from build123d import *

# Parameters (mm, degrees)
BOSS_EXTRUDE1_DEPTH = 1.5
CHAMFER1_SIZE2      = 1.091910703
CHAMFER1_SIZE       = 3
SKETCH3_W           = 60
SKETCH3_H           = 48.2
CUT_EXTRUDE2_DEPTH  = 69.98434605
FILLET1_R           = 5


with BuildPart() as part:
    # Sketch1 → Boss-Extrude1 (new, symmetric)
    with BuildSketch(Plane.XY):
        Polygon((-45, 0), (45, 0), (41, 52.2), (-41, 52.2), align=None)
    extrude(amount=BOSS_EXTRUDE1_DEPTH, both=True)

    # Chamfer1
    chamfer1_edges = [part.edges().sort_by_distance(p)[0] for p in [
        (0, 0, -1.5),
    ]]
    chamfer1_side = [part.faces().sort_by_distance(p)[0] for p in [
        (0, 0, -1.478161786),
    ]]
    chamfer(chamfer1_edges, length=CHAMFER1_SIZE - 0.0001, length2=CHAMFER1_SIZE2 - 0.0001, reference=chamfer1_side[0])  # a hair under: the kernel refuses the full size

    # Sketch3 → Cut-Extrude2 (cut, through all)
    with BuildSketch(Plane.XY.offset(1.5)):
        with Locations((-15, 24.1)):
            Rectangle(SKETCH3_W, SKETCH3_H)
    extrude(amount=-CUT_EXTRUDE2_DEPTH, mode=Mode.SUBTRACT)

    # Fillet1
    fillet1_edges = [part.edges().sort_by_distance(p)[0] for p in [
        (15, 48.2, 0),
    ]]
    fillet(fillet1_edges, radius=FILLET1_R)


solid = part.part
Here's how the part is built. I have some questions about the finished solid (model axes, mm). A direction names the side the tool comes from. Give positions to 0.01 mm unless a question says otherwise; leave off trailing zeros. Loops run counter-clockwise (first coordinate to the right, second up) from the corner with the lowest first, then second, coordinate; pieces in that order, holes last. Notation, with made-up numbers: (-11.5, 78.25) -> (3.5, 78.25) arc R30 ccw to (3.5, 114.25) -> close; hole circle Ø3 at (24, 71.25). An arc over 180 degrees is marked (long way). One line per item, written item: value.
Q1. Suppose I cut it at B-B on x = 0.5. Please give me the cut outline in (y, z), then the cut area to 3 significant figures.
Answers follow:
outline: (48.2, -1.5) -> (52.2, -1.5) -> (52.2, 1.5) -> (48.2, 1.5) -> close
area: 12.0 mm^2
Q2. If I drill on line 1 along Y through (x, z) = (-31.5, -1.2); line 2 along X through (y, z) = (29.5, 0); line 3 along X through (y, z) = (8.5, 0.85), over which ranges is the centre line in solid material (lowest first)?
Answers follow:
line 1: 48.2 to 52.2
line 2: 15 to 42.74
line 3: 15 to 44.35
Q3. I'm going to push flat-ended pins straight in: pin 1 Ø0.9 at (y, z) = (15.5, 0.5) entering from -X; pin 2 Ø1 at (x, z) = (-3.5, -0.5) entering from -Y; pin 3 Ø1 at (y, z) = (44.5, -1) entering from -X. Where does each tip first touch, or does it pass through?
Answers follow:
pin 1: x = 15
pin 2: y = 48.2
pin 3: x = 14.66
Q4. Suppose I cut it at A-A on z = 0.85. Please give me the cut outline in (x, y).
Answers follow:
outline: (-41.31, 48.2) -> (10, 48.2) arc R5 cw to (15, 43.2) -> (15, 0.24) -> (44.98, 0.24) -> (41, 52.2) -> (-41, 52.2) -> close
Q5. Suppose I cut it at C-C on y = 41. Please give me the cut outline in (x, z), then the cut area to 3 significant figures.
Answers follow:
outline: (15, -1.5) -> (41.86, -1.5) -> (41.86, 1.5) -> (15, 1.5) -> close
area: 80.6 mm^2
Q6. On a 3-axis mill with a long thin cutter (end or side, diameter ignored), from which of +Z, -Z, +X, -X, +Y, -Y can I reach the whole of each face in a straight line? I mean faces 1 (the face through (-16, 48.2, 0)), 2 (the face through (-41.15, 50.23, 0.02)). Say none if no direction works.
Answers follow:
face 1: +Z, -Z, -X, -Y
face 2: +Z, -Z, -X, +Y
